Autodesk Inventor part; units mm, degrees
ref_plane "YZ Plane" through (0, 0, 0) normal (1, 0, 0) x (0, 1, 0)
ref_plane "XZ Plane" through (0, 0, 0) normal (0, 1, 0) x (-1, 0, 0)
ref_plane "XY Plane" through (0, 0, 0) normal (0, 0, 1) x (1, 0, 0)
sketch "Sketch1" plane through (0, 0, 0) normal (0, 0, 1) x (1, 0, 0)
  line L0 (0, 0) -> (22, 0)
  line L1 (22, 0) -> (22, 22)
  line L2 (22, 22) -> (0, 22)
  line L3 (0, 22) -> (0, 0)
  dimension "d0" = 22
  dimension "d1" = 22
extrude "Extrusion1" add sketch "Sketch1" along normal blind 5
sketch "Sketch2" plane through (0, 0, 5) normal (0, 0, 1) x (1, 0, 0)
  circle A0 centre (3.5, 18.5) radius 1.5
  circle A1 centre (18.5, 18.5) radius 1.5
  line L0 (0, 22) -> (0, 0)
  line L1 (22, 22) -> (0, 22)
  circle A2 centre (3.5, 3.5) radius 1.5
  line L2 (0, 0) -> (22, 0)
  circle A3 centre (18.5, 3.5) radius 1.5
  line L3 (22, 0) -> (22, 22)
  dimension "d4" = 3
  dimension "d5" = 3
  dimension "d6" = 3.5
  dimension "d7" = 15
  dimension "d8" = 3.5
  dimension "d9" = 3.5
  dimension "d10" = 3
  dimension "d11" = 3.5
  dimension "d12" = 3.5
  dimension "d13" = 3
  dimension "d14" = 3.5
  dimension "d15" = 3.5
hole "Hole1" at (3.5, 18.5, 5) at (18.5, 18.5, 5) at (18.5, 3.5, 5) at (3.5, 3.5, 5) direction (0, 0, -1) diameter 3.2 end through all counterbore diameter 5.7 counterbore depth 3.4
sketch "Sketch3" plane through (0, 0, 5) normal (0, 0, 1) x (1, 0, 0)
  circle A0 centre (7.5, 7.5) radius 1.5
  line L0 (0, 22) -> (0, 0)
  line L1 (0, 0) -> (22, 0)
  circle A1 centre (7.5, 14.5) radius 1.5
  circle A2 centre (14.5, 7.5) radius 1.5
  circle A3 centre (14.5, 14.5) radius 1.5
  dimension "d23" = 3
  dimension "d24" = 7.5
  dimension "d25" = 7.5
  dimension "d33" = 3
  dimension "d34" = 3
  dimension "d35" = 3
  dimension "d36" = 7
  dimension "d37" = 7
  dimension "d38" = 7
  dimension "d39" = 0
  dimension "d40" = 7.5
  dimension "d41" = 7
hole "Hole2" at (7.5, 7.5, 5) at (7.5, 14.5, 5) at (14.5, 7.5, 5) at (14.5, 14.5, 5) direction (0, 0, -1) diameter 2.156 end through all
sketch "Sketch7" plane through (0, 0, 5) normal (0, 0, 1) x (1, 0, 0)
  circle A0 centre (11, 11) radius 1.5
  line L0 (22, 22) -> (0, 22)
  line L1 (22, 0) -> (22, 22)
  point P0 (0, 0)
  dimension "d64" = 3
  dimension "d65" = 11
  dimension "d66" = 11
hole "Hole5" at (11, 11, 5) direction (0, 0, -1) diameter 3.05 end through all
sketch "Sketch8" plane through (0, 0, 0) normal (0, 0, -1) x (-1, 0, 0)
  circle A0 centre (-11, 11) radius 1.525
  circle A1 centre (-11, 11) radius 2.45
  point P0 (0, 0)
  dimension "d74" = 4.9
hole "Hole6" at (11, 11, 0) direction (0, 0, 1) diameter 4.9 depth 3.05 tip angle 118
equation "\"d21\" = Thickness"
equation "\"d23\" = d35"
equation "\"d33\" = d35"
equation "\"d34\" = d35"
equation "\"d36\" = d38"
equation "\"d37\" = d38"
equation "\"d40\" = d25"
equation "\"BendRadius\" = Thickness"
equation "\"BendReliefWidth\" = Thickness"
equation "\"BendReliefDepth\" = 0.5 * Thickness"
equation "\"CornerReliefSize\" = 4 * Thickness"
equation "\"MinimumRemnant\" = 2 * Thickness"
equation "\"TransitionRadius\" = BendRadius"
equation "\"JacobiRadiusSize\" = BendRadius"
equation "\"GapSize\" = Thickness"
properties part number "sample holder mount on PI_V_522_v2"
Source: CAD feature listing. Evaluate the final solid. Frame: model axes, mm. A direction names the side the tool comes from. Round coordinates to 2 decimals unless told otherwise and drop trailing zeros. Loops run counter-clockwise (first coordinate to the right, second up) from the corner with the lowest first, then second, coordinate; pieces in that order, holes last.
1. Access query for faces 1 (the flat face through (20, 2, 1.6)), 2 (the flat face through (13, 11, 5)). Directions: +Z, -Z, +X, -X, +Y, -Y. A direction counts if a zero-diameter tool reaches every point of the face in a straight line with its end or side. Return the directions, or none.
2. Section query C-C on z = 4.15. Give the number of separate pieces and of enclosed holes in the cut face, and give its area (3 significant figures).
3. Section query A-A on y = 18.5. Output: boundary loops of the cut face in (x, z), and give its area (3 significant figures).
4. Ray query, L1, parallel to X at y = 3.5, z = 0.7; L2, parallel to X at y = 3.5, z = 2.15. Return the intervals inside material, ascending.
5. Section query D-D on y = 11. Output: boundary loops of the cut face in (x, z) (3 decimals), and give its area (3 significant figures).
6. Section query B-B on x = 14.5. Output: boundary loops of the cut face in (y, z).
7. Mould query, pull axis X, two halves, no side actions, for faces 3 (the flat face through (0, 11, 2)), 4 (the flat face through (5, 17, 1.6)), 5 (the flat face through (11, 0, 2)). Classes: released by +X, released by -X, zero draft, split by the parting line, or undercut.
8. Contact query for a flat-ended pin moving along its axis: pin 1 (5 mm diameter, centred on x = 18.5, y = 18.5, fed in from +Z). Output: stop coordinate, or through.
Answers below:
1. face 1: +Z
1. face 2: +Z, +X, -X, +Y, -Y
2. separate pieces: 1
2. enclosed holes: 9
2. area: 360 mm2
3. outline: (0, 0) - (1.9, 0) - (1.9, 1.6) - (0.65, 1.6) - (0.65, 5) - (0, 5) - close; (5.1, 0) - (16.9, 0) - (16.9, 1.6) - (15.65, 1.6) - (15.65, 5) - (6.35, 5) - (6.35, 1.6) - (5.1, 1.6) - close; (20.1, 0) - (22, 0) - (22, 5) - (21.35, 5) - (21.35, 1.6) - (20.1, 1.6) - close
3. area: 61.0 mm2
4. L1: x = 0 to 1.9, 5.1 to 16.9, 20.1 to 22
4. L2: x = 0 to 0.65, 6.35 to 15.65, 21.35 to 22
5. outline: (0, 0) - (8.55, 0) - (8.55, 3.05) - (9.475, 3.606) - (9.475, 5) - (0, 5) - close; (12.525, 3.606) - (13.45, 3.05) - (13.45, 0) - (22, 0) - (22, 5) - (12.525, 5) - close
5. area: 88.6 mm2
6. outline: (0, 0) - (6.42, 0) - (6.42, 5) - (0, 5) - close; (8.58, 0) - (13.42, 0) - (13.42, 5) - (8.58, 5) - close; (15.58, 0) - (22, 0) - (22, 5) - (15.58, 5) - close
7. face 3: released by -X
7. face 4: undercut
7. face 5: zero draft
8. pin 1: stops at z = 1.6
